Geometry: see drawing. Coordinates: mm, zero at the bounding-box minimum. Coordinates: 2 decimals unless noted, no trailing zeros. Order: outer loops, then holes, each group sorted by start corner. A loop starts at its lowest first (then second) coordinate and runs counter-clockwise, first axis right, second up. Notation, with made-up numbers: M 66,27 L 71,27 A16 cw 71,41 Z; hole C 52.25,48.25 d11. An arc over 180 degrees is marked long. Answer in a Markdown table with one row per item.
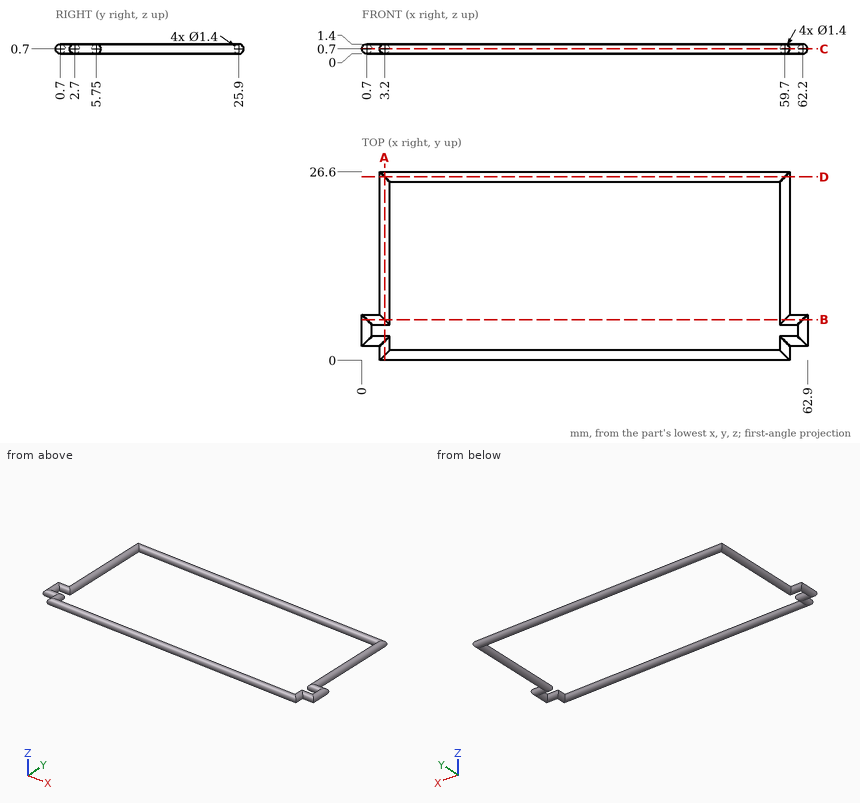
1) Contact query for a flat-ended pin moving along its axis: pin 1 (4 mm diameter, centred on x = 56.5, y = 11, fed in from -Z). Output: stop coordinate, or through.
Resolved:
| item | result |
|---|---|
| pin 1 | passes through |
2) Cut plane B-B, the plane y = 5.75. Output: boundary loops of the cut face in (x, z), and give its area (3 significant figures).
Resolved:
| item | result |
|---|---|
| outline | M 0.7,0 L 3.2,0 A0.7 ccw 3.2,1.4 L 0.7,1.4 A0.7 ccw Z; M 59.7,0 L 62.2,0 A0.7 ccw 62.2,1.4 L 59.7,1.4 A0.7 ccw Z |
| area | 10.1 mm2 |
3) Material intervals for probe 1 along X at (y, z) = (12.75, 0.65); probe 2 along Y at (x, z) = (6.5, 0.6); probe 3 along Y at (x, z) = (22, 0.25), sorted ascending.
Resolved:
| item | result |
|---|---|
| probe 1 | x = 2.5 to 3.9, 59 to 60.4 |
| probe 2 | y = 0.01 to 1.39, 25.21 to 26.59 |
| probe 3 | y = 0.16 to 1.24, 25.36 to 26.44 |
4) Cut plane C-C, the plane z = 0.7. Output: boundary loops of the cut face in (x, y), and give its area (3 significant figures).
Resolved:
| item | result |
|---|---|
| outline | M 0,2 L 2.5,2 L 2.5,0 L 60.4,0 L 60.4,2 L 62.9,2 L 62.9,6.45 L 60.4,6.45 L 60.4,26.6 L 2.5,26.6 L 2.5,6.45 L 0,6.45 Z; hole M 1.4,3.4 L 3.9,3.4 L 3.9,1.4 L 59,1.4 L 59,3.4 L 61.5,3.4 L 61.5,5.05 L 59,5.05 L 59,25.2 L 3.9,25.2 L 3.9,5.05 L 1.4,5.05 Z |
| area | 243 mm2 |
5) Cut plane A-A, the plane x = 3.2. Output: boundary loops of the cut face in (y, z).
Resolved:
| item | result |
|---|---|
| outline | M 0.7,0 L 2.7,0 A0.7 ccw 2.7,1.4 L 0.7,1.4 A0.7 ccw Z; M 5.75,0 L 25.9,0 A0.7 ccw 25.9,1.4 L 5.75,1.4 A0.7 ccw Z |
6) Cut plane D-D, the plane y = 25.9. Output: boundary loops of the cut face in (x, z).
Resolved:
| item | result |
|---|---|
| outline | M 3.2,0 L 59.7,0 A0.7 ccw 59.7,1.4 L 3.2,1.4 A0.7 ccw Z |
